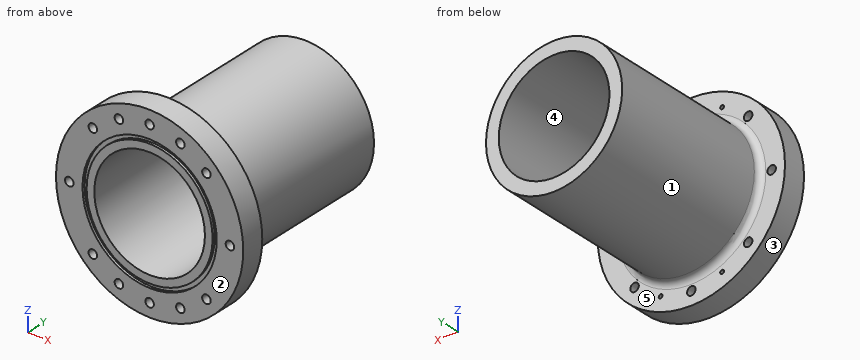
from build123d import *

# Parameters (mm, degrees)
SKETCH2_R               = 50.8
SKETCH2_R_2             = 41.275
BASE_CYLINDER_DEPTH     = 292.1
SKETCH3_R               = 69.85
SKETCH3_R_2             = 41.275
AFT_FLANGE_DEPTH        = 17.78
SKETCH4_R               = 69.85
SKETCH4_R_2             = 41.275
FORWARD_FLANGE_DEPTH    = 17.78
SKETCH6_R               = 50.0761
SKETCH6_R_2             = 47.0027
O_RING_SLOT_1_DEPTH     = 1.9812
SKETCH7_R               = 50.0761
SKETCH7_R_2             = 47.0027
O_RING_SLOT_2_DEPTH     = 1.9812
SKETCH8_R               = 3.175
CUT_EXTRUDE4_DEPTH      = 1
CUT_EXTRUDE4_DEPTH_BACK = 293.1
FILLET1_R               = 4.7625
SKETCH9_R               = 3.175
CUT_EXTRUDE5_DEPTH      = 7.62
SKETCH10_R              = 3.175
CUT_EXTRUDE6_DEPTH      = 7.62
CUT_EXTRUDE7_REACH      = 286.48
SKETCH11_R              = 1.4097
CUT_EXTRUDE8_REACH      = 286.48
SKETCH12_R              = 1.4097
SKETCH13_R              = 2.3114
CUT_EXTRUDE10_DEPTH     = 6.35
SKETCH14_R              = 2.3114
CUT_EXTRUDE11_DEPTH     = 6.35
SKETCH18_R              = 69.85
CUT_EXTRUDE13_DEPTH     = 146.05


with BuildPart() as part:
    # Sketch2 → Base Cylinder (new body)
    with BuildSketch(Plane(origin=(0, 0, 0), x_dir=(1, 0, 0), z_dir=(0, 1, 0))):
        Circle(SKETCH2_R)
        Circle(SKETCH2_R_2, mode=Mode.SUBTRACT)
    extrude(amount=BASE_CYLINDER_DEPTH)

    # Sketch3 → Aft Flange (add)
    with BuildSketch(Plane.XZ):
        Circle(SKETCH3_R)
        Circle(SKETCH3_R_2, mode=Mode.SUBTRACT)
    extrude(amount=-AFT_FLANGE_DEPTH)

    # Sketch4 → Forward Flange (add)
    with BuildSketch(Plane(origin=(0, 292.1, 0), x_dir=(1, 0, 0), z_dir=(0, 1, 0))):
        Circle(SKETCH4_R)
        Circle(SKETCH4_R_2, mode=Mode.SUBTRACT)
    extrude(amount=-FORWARD_FLANGE_DEPTH)

    # Sketch6 → O-Ring Slot 1 (cut)
    with BuildSketch(Plane.XZ):
        Circle(SKETCH6_R)
        Circle(SKETCH6_R_2, mode=Mode.SUBTRACT)
    extrude(amount=-O_RING_SLOT_1_DEPTH, mode=Mode.SUBTRACT)

    # Sketch7 → O-Ring Slot 2 (cut)
    with BuildSketch(Plane(origin=(0, 292.1, 0), x_dir=(1, 0, 0), z_dir=(0, 1, 0))):
        Circle(SKETCH7_R)
        Circle(SKETCH7_R_2, mode=Mode.SUBTRACT)
    extrude(amount=-O_RING_SLOT_2_DEPTH, mode=Mode.SUBTRACT)

    # Sketch8 → Cut-Extrude4 (cut, two sides)
    with BuildSketch(Plane.XZ) as cut_extrude4_sk:
        with Locations((-59.9186, 0)):
            Circle(SKETCH8_R)
        with Locations((-42.368848379, 42.368848379)):
            Circle(SKETCH8_R)
        with Locations((0, 59.9186)):
            Circle(SKETCH8_R)
        with Locations((42.368848379, 42.368848379)):
            Circle(SKETCH8_R)
        with Locations((59.9186, 0)):
            Circle(SKETCH8_R)
        with Locations((42.368848379, -42.368848379)):
            Circle(SKETCH8_R)
        with Locations((0, -59.9186)):
            Circle(SKETCH8_R)
        with Locations((-42.368848379, -42.368848379)):
            Circle(SKETCH8_R)
    extrude(amount=CUT_EXTRUDE4_DEPTH, mode=Mode.SUBTRACT)
    extrude(cut_extrude4_sk.sketch, amount=-CUT_EXTRUDE4_DEPTH_BACK, mode=Mode.SUBTRACT)

    # Fillet1
    fillet1_edges = [part.edges().sort_by_distance(p)[0] for p in [
        (-50.8, 17.78, 0),
        (-50.8, 274.32, 0),
    ]]
    fillet(fillet1_edges, radius=FILLET1_R)

    # Sketch9 → Cut-Extrude5 (cut)
    with BuildSketch(Plane(origin=(0, 292.1, 0), x_dir=(1, 0, 0), z_dir=(0, 1, 0))):
        with Locations((-22.929855511, 55.357568157)):
            Circle(SKETCH9_R)
        with Locations((22.929855511, -55.357568157)):
            Circle(SKETCH9_R)
        with Locations((22.929855511, 55.357568157)):
            Circle(SKETCH9_R)
        with Locations((-22.929855511, -55.357568157)):
            Circle(SKETCH9_R)
    extrude(amount=-CUT_EXTRUDE5_DEPTH, mode=Mode.SUBTRACT)

    # Sketch10 → Cut-Extrude6 (cut)
    with BuildSketch(Plane.XZ):
        with Locations((-22.929855511, 55.357568157)):
            Circle(SKETCH10_R)
        with Locations((22.929855511, -55.357568157)):
            Circle(SKETCH10_R)
        with Locations((22.929855511, 55.357568157)):
            Circle(SKETCH10_R)
        with Locations((-22.929855511, -55.357568157)):
            Circle(SKETCH10_R)
    extrude(amount=-CUT_EXTRUDE6_DEPTH, mode=Mode.SUBTRACT)

    # Sketch11 → Cut-Extrude7 (cut, up to next)
    with BuildSketch(Plane(origin=(0, 284.48, 0), x_dir=(1, 0, 0), z_dir=(0, 1, 0)), mode=Mode.PRIVATE) as cut_extrude7_sk1:
        with Locations((-22.929855511, 55.357568157)):
            Circle(SKETCH11_R)
    cut_extrude7_tool1 = extrude(cut_extrude7_sk1.sketch, amount=-CUT_EXTRUDE7_REACH, mode=Mode.PRIVATE) & part.part
    add(cut_extrude7_tool1.solids().sort_by_distance((-22.929856, 284.48, -55.357568))[0], mode=Mode.SUBTRACT)
    # Sketch11 → Cut-Extrude7 (cut, up to next)
    with BuildSketch(Plane(origin=(0, 284.48, 0), x_dir=(1, 0, 0), z_dir=(0, 1, 0)), mode=Mode.PRIVATE) as cut_extrude7_sk2:
        with Locations((22.929855511, 55.357568157)):
            Circle(SKETCH11_R)
    cut_extrude7_tool2 = extrude(cut_extrude7_sk2.sketch, amount=-CUT_EXTRUDE7_REACH, mode=Mode.PRIVATE) & part.part
    add(cut_extrude7_tool2.solids().sort_by_distance((22.929856, 284.48, -55.357568))[0], mode=Mode.SUBTRACT)
    # Sketch11 → Cut-Extrude7 (cut, up to next)
    with BuildSketch(Plane(origin=(0, 284.48, 0), x_dir=(1, 0, 0), z_dir=(0, 1, 0)), mode=Mode.PRIVATE) as cut_extrude7_sk3:
        with Locations((-22.929855511, -55.357568157)):
            Circle(SKETCH11_R)
    cut_extrude7_tool3 = extrude(cut_extrude7_sk3.sketch, amount=-CUT_EXTRUDE7_REACH, mode=Mode.PRIVATE) & part.part
    add(cut_extrude7_tool3.solids().sort_by_distance((-22.929856, 284.48, 55.357568))[0], mode=Mode.SUBTRACT)
    # Sketch11 → Cut-Extrude7 (cut, up to next)
    with BuildSketch(Plane(origin=(0, 284.48, 0), x_dir=(1, 0, 0), z_dir=(0, 1, 0)), mode=Mode.PRIVATE) as cut_extrude7_sk4:
        with Locations((22.929855511, -55.357568157)):
            Circle(SKETCH11_R)
    cut_extrude7_tool4 = extrude(cut_extrude7_sk4.sketch, amount=-CUT_EXTRUDE7_REACH, mode=Mode.PRIVATE) & part.part
    add(cut_extrude7_tool4.solids().sort_by_distance((22.929856, 284.48, 55.357568))[0], mode=Mode.SUBTRACT)

    # Sketch12 → Cut-Extrude8 (cut, up to next)
    with BuildSketch(Plane.XZ.offset(-7.62), mode=Mode.PRIVATE) as cut_extrude8_sk1:
        with Locations((-22.929855511, 55.357568157)):
            Circle(SKETCH12_R)
    cut_extrude8_tool1 = extrude(cut_extrude8_sk1.sketch, amount=-CUT_EXTRUDE8_REACH, mode=Mode.PRIVATE) & part.part
    add(cut_extrude8_tool1.solids().sort_by_distance((-22.929856, 7.62, 55.357568))[0], mode=Mode.SUBTRACT)
    # Sketch12 → Cut-Extrude8 (cut, up to next)
    with BuildSketch(Plane.XZ.offset(-7.62), mode=Mode.PRIVATE) as cut_extrude8_sk2:
        with Locations((22.929855511, 55.357568157)):
            Circle(SKETCH12_R)
    cut_extrude8_tool2 = extrude(cut_extrude8_sk2.sketch, amount=-CUT_EXTRUDE8_REACH, mode=Mode.PRIVATE) & part.part
    add(cut_extrude8_tool2.solids().sort_by_distance((22.929856, 7.62, 55.357568))[0], mode=Mode.SUBTRACT)
    # Sketch12 → Cut-Extrude8 (cut, up to next)
    with BuildSketch(Plane.XZ.offset(-7.62), mode=Mode.PRIVATE) as cut_extrude8_sk3:
        with Locations((-22.929855511, -55.357568157)):
            Circle(SKETCH12_R)
    cut_extrude8_tool3 = extrude(cut_extrude8_sk3.sketch, amount=-CUT_EXTRUDE8_REACH, mode=Mode.PRIVATE) & part.part
    add(cut_extrude8_tool3.solids().sort_by_distance((-22.929856, 7.62, -55.357568))[0], mode=Mode.SUBTRACT)
    # Sketch12 → Cut-Extrude8 (cut, up to next)
    with BuildSketch(Plane.XZ.offset(-7.62), mode=Mode.PRIVATE) as cut_extrude8_sk4:
        with Locations((22.929855511, -55.357568157)):
            Circle(SKETCH12_R)
    cut_extrude8_tool4 = extrude(cut_extrude8_sk4.sketch, amount=-CUT_EXTRUDE8_REACH, mode=Mode.PRIVATE) & part.part
    add(cut_extrude8_tool4.solids().sort_by_distance((22.929856, 7.62, -55.357568))[0], mode=Mode.SUBTRACT)

    # Sketch13 → Cut-Extrude10 (cut)
    with BuildSketch(Plane(origin=(-69.85, 0, 0), x_dir=(0, 0, -1), z_dir=(1, 0, 0))):
        with Locations((0, 283.21)):
            Circle(SKETCH13_R)
    extrude(amount=CUT_EXTRUDE10_DEPTH, mode=Mode.SUBTRACT)

    # Sketch14 → Cut-Extrude11 (cut)
    with BuildSketch(Plane(origin=(69.85, 0, 0), x_dir=(0, 0, -1), z_dir=(1, 0, 0))):
        with Locations((0, 283.21)):
            Circle(SKETCH14_R)
    extrude(amount=-CUT_EXTRUDE11_DEPTH, mode=Mode.SUBTRACT)

    # Sketch18 → Cut-Extrude13 (cut)
    with BuildSketch(Plane(origin=(0, 292.1, 0), x_dir=(1, 0, 0), z_dir=(0, 1, 0))):
        Circle(SKETCH18_R)
    extrude(amount=-CUT_EXTRUDE13_DEPTH, mode=Mode.SUBTRACT)


solid = part.part
The listing builds one solid part. Answer for the finished solid, in the listing's coordinates (mm). Face numbers are marked on the shaded views. A direction names the side the tool comes from. Give positions to 0.01 mm unless a question says otherwise; leave off trailing zeros. Write each loop counter-clockwise with the first axis right and the second up, starting at its lowest first coordinate (ties: lowest second). Pieces come first, ordered by that corner, then holes.
Item 1: Section C-C, the plane y = 100.5 is taken. Write down the section's boundary in (x, z) (3 decimals), plus the area to 3 significant figures.
Item 2: Flat-ended cylindrical pins translate along their axes: P1, Ø5, axis at x = -22.93, z = 55.36, coming from the +Y side; P2, Ø10, axis at x = -11, y = 130.5, coming from the -Z side; P3, Ø5, axis at y = 125.5, z = 15, coming from the +X side. Find the tip coordinate at first contact, or state that the pin passes through.
Item 3: Which of the six approach directions +Z, -Z, +X, -X, +Y, -Y give full straight-line access (tool end or side, diameter ignored) to the marked faces 1 and 2?
Item 4: Section A-A, the plane z = 0 is taken. Count the separate pieces of the cut face and the enclosed holes in it, plus the area to 3 significant figures.
Item 5: Determine the mould class of the marked faces 3, 4 and 5 for opening direction X: released by +X, released by -X, zero draft, split by the parting line, or undercut.
Item 6: Find the intervals of material crossed by line 1 along Z through (x, y) = (0, 0.8) (3 decimals); line 2 along Z through (x, y) = (0, 10) (3 decimals); line 3 along X through (y, z) = (140, 1.5), in increasing order.
Completed:
1. outline: circle Ø101.6 at (0, 0); hole circle Ø82.55 at (0, 0)
1. area: 2,760 mm2
2. P1: stops at y = 17.78
2. P2: stops at z = -50.44
2. P3: stops at x = 49.24
3. face 1: +Y
3. face 2: +Z, -Z, +X, -X, -Y
4. separate pieces: 4
4. enclosed holes: 0
4. area: 3,230 mm2
5. face 3: split by the parting line
5. face 4: undercut
5. face 5: zero draft
6. line 1: z = -69.85 to -63.094, -56.744 to -50.076, -47.003 to -41.275, 41.275 to 47.003, 50.076 to 56.744, 63.094 to 69.85
6. line 2: z = -69.85 to -63.094, -56.744 to -41.275, 41.275 to 56.744, 63.094 to 69.85
6. line 3: x = -50.78 to -41.25, 41.25 to 50.78
